Could you check a few things on this model? Use its own coordinates, in mm. Round coordinates to 2 decimals unless told otherwise and drop trailing zeros. Order: outer loops, then holes, each group sorted by start corner. A loop starts at its lowest first (then second) coordinate and runs counter-clockwise, first axis right, second up. Notation, with made-up numbers: (67.25, 55) -> (114.25, 55) arc R7 cw to (114.25, 62) -> close; hole circle Ø11 at (61, 74). An arc over 180 degrees is marked (long way). One line per question, with ' | ' between items.
Autodesk Inventor part; units mm, degrees
ref_plane "YZ Plane" through (0, 0, 0) normal (1, 0, 0) x (0, 1, 0)
ref_plane "XZ Plane" through (0, 0, 0) normal (0, 1, 0) x (-1, 0, 0)
ref_plane "XY Plane" through (0, 0, 0) normal (0, 0, 1) x (1, 0, 0)
sketch "Sketch1" plane through (0, 0, 0) normal (0, 0, 1) x (1, 0, 0)
  line L0 (0, 0) -> (0, 12.3467)
  line L1 (0, 0) -> (3, 0)
  line L2 (3, 0) -> (3, 1.5)
  line L3 (3, 1.5) -> (2.85, 1.5)
  line L4 (2.85, 1.5) -> (2.85, 3.2)
  line L5 (2.85, 3.2) -> (5.4, 3.2)
  line L6 (5.4, 3.2) -> (5.4, 6.4)
  line L7 (5.4, 6.4) -> (0, 6.4)
  line L8 (0, 0) -> (0, 6.4)
  dimension "d1" = 5.7
  dimension "d2" = 6
  dimension "d3" = 10.8
  dimension "d4" = 1.5
  dimension "d6" = 6.4
  dimension "d7" = 3.2
revolve "Revolution1" add sketch "Sketch1" angle 360 about axis through (0, 0, 0) along (0, 1, 0)
fillet "Fillet1" radius 1.6 1 edges at (-2.85, 3.2, 0)
chamfer "Chamfer1" distance 0.2 angle 45 2 edges at (-5.4, 6.4, 0) (-5.4, 3.2, 0)
hole "Hole1" at (0, 6.4, 0) direction (0, -1, 0) diameter 2.459 end through all
properties part number "Bed Thumb Screw" material "Stainless Steel"
1. If we mould it in two halves opening along Y, with no side actions, what happens to faces 1 (the face through (-3, 1, 0)), 2 (the face through (1, 0, 1)), 3 (the face through (1, 6.4, 1))? For each: pulls with the +Y half, pulls with the -Y half, needs draft (parallel to the pull), parting line crosses it, or undercut.
From the geometry:
face 1: needs draft | face 2: pulls with the -Y half | face 3: pulls with the +Y half
2. I need wall thicknesses on probe 1 along X at (y, z) = (5.25, 0); probe 2 along Y at (x, z) = (1.25, -4.5). Which ranges of each line are inside material? Lowest first, please.
From the geometry:
probe 1: x = -5.4 to -1.23, 1.23 to 5.4 | probe 2: y = 3.2 to 6.4
3. I want a section at D-D on y = 0.75. List the corners of the cut face in (x, z) for me.
From the geometry:
outline: circle Ø6 at (0, 0); hole circle Ø2.46 at (0, 0)
4. I want a section at A-A on z = 0. List the corners of the cut face in (x, y) for me, and give its area (3 significant figures).
From the geometry:
outline: (-5.4, 3.4) -> (-5.2, 3.2) -> (-4.45, 3.2) arc R1.6 cw to (-2.85, 1.6) -> (-2.85, 1.5) -> (-3, 1.5) -> (-3, 0) -> (-1.23, 0) -> (-1.23, 6.4) -> (-5.2, 6.4) -> (-5.4, 6.2) -> close; (1.23, 0) -> (3, 0) -> (3, 1.5) -> (2.85, 1.5) -> (2.85, 1.6) arc R1.6 cw to (4.45, 3.2) -> (5.2, 3.2) -> (5.4, 3.4) -> (5.4, 6.2) -> (5.2, 6.4) -> (1.23, 6.4) -> close | area: 38.5 mm²
5. I want a section at B-B on x = 0. List the corners of the cut face in (y, z) for me.
From the geometry:
outline: (0, -3) -> (1.5, -3) -> (1.5, -2.85) -> (1.6, -2.85) arc R1.6 cw to (3.2, -4.45) -> (3.2, -5.2) -> (3.4, -5.4) -> (6.2, -5.4) -> (6.4, -5.2) -> (6.4, -1.23) -> (0, -1.23) -> close; (0, 1.23) -> (6.4, 1.23) -> (6.4, 5.2) -> (6.2, 5.4) -> (3.4, 5.4) -> (3.2, 5.2) -> (3.2, 4.45) arc R1.6 cw to (1.6, 2.85) -> (1.5, 2.85) -> (1.5, 3) -> (0, 3) -> close
6. I'm going to push flat-ended pins straight in: pin 1 (6 mm diameter, centred on x = -2.5, z = -1.5, fed in from -Y); pin 2 (1 mm diameter, centred on x = -3, y = 2, fed in from -Z); pin 3 (2 mm diameter, centred on x = 0, z = 0, fed in from -Y); pin 4 (1.5 mm diameter, centred on x = -4, z = -3, fed in from -Y). Where does each tip first touch, or does it pass through?
From the geometry:
pin 1: stops at y = 0 | pin 2: stops at z = -1.53 | pin 3: passes through | pin 4: stops at y = 3.19
7. I want a section at C-C on y = 5.5. List the corners of the cut face in (x, z) for me.
From the geometry:
outline: circle Ø10.8 at (0, 0); hole circle Ø2.46 at (0, 0)
